Here's how the part is built. I have some questions about the finished solid (model axes, mm). Give positions to 0.01 mm unless a question says otherwise; leave off trailing zeros. Write each loop counter-clockwise with the first axis right and the second up, starting at its lowest first coordinate (ties: lowest second). Pieces come first, ordered by that corner, then holes. Notation, with made-up numbers: (-15, 55) - (33, 55) arc R33 ccw to (33, 85) - close; hole circle Ø7 at (17.5, -35). An arc over 180 degrees is marked (long way). Use a Markdown table: item, result.
```python
from build123d import *

# Parameters (mm, degrees)
EXTRUDE_1_DEPTH     = 5
SKETCH_2_R          = 1.25
CUT_EXTRUDE_1_DEPTH = 5


with BuildPart() as part:
    # 草图1 → 凸台-拉伸1 (new body, symmetric)
    with BuildSketch(Plane(origin=(0, 0, 0), x_dir=(1, 0, 0), z_dir=(0, 1, 0))):
        Polygon((0, -2.598076211), (2.25, -1.299038106), (2.25, 1.299038106), (0, 2.598076211), (-2.25, 1.299038106), (-2.25, -1.299038106), align=None)
    extrude(amount=EXTRUDE_1_DEPTH, both=True)

    # 草图2 → 切除-拉伸1 (cut)
    with BuildSketch(Plane(origin=(0, 5, 0), x_dir=(1, 0, 0), z_dir=(0, 1, 0))):
        Circle(SKETCH_2_R)
    extrude(amount=-CUT_EXTRUDE_1_DEPTH, mode=Mode.SUBTRACT)


solid = part.part
```
Item 1: If we section it at D-D, the plane x = -1.4: Write out the boundary of the cut face in (y, z), plus the area to 3 significant figures.
Values:
| item | result |
|---|---|
| outline | (-5, -1.79) - (5, -1.79) - (5, 1.79) - (-5, 1.79) - close |
| area | 35.8 mm2 |
Item 2: If we section it at B-B, the plane z = -1: Write out the boundary of the cut face in (x, y), plus the area to 3 significant figures.
Values:
| item | result |
|---|---|
| outline | (-2.25, -5) - (2.25, -5) - (2.25, 5) - (0.75, 5) - (0.75, 0) - (-0.75, 0) - (-0.75, 5) - (-2.25, 5) - close |
| area | 37.5 mm2 |
Item 3: I need wall thicknesses on line 1 along X through (y, z) = (2.2, 0); line 2 along X through (y, z) = (3.25, -0.5); line 3 along Y through (x, z) = (-0.45, 0.35). Which ranges of each line are inside material? Lowest first, please. Write a range as [from, to].
Values:
| item | result |
|---|---|
| line 1 | x = [-2.25, -1.25], [1.25, 2.25] |
| line 2 | x = [-2.25, -1.15], [1.15, 2.25] |
| line 3 | y = [-5, 0] |
Item 4: If we section it at C-C, the plane x = 1.15: Write out the boundary of the cut face in (y, z), plus the area to 3 significant figures.
Values:
| item | result |
|---|---|
| outline | (-5, -1.93) - (5, -1.93) - (5, -0.49) - (0, -0.49) - (0, 0.49) - (5, 0.49) - (5, 1.93) - (-5, 1.93) - close |
| area | 33.8 mm2 |
Item 5: Thinking about a two-plate mould opening in Z: for faces 1 (the cylindrical face through (-0.27, 2.54, 1.22)), 2 (the flat face through (0, 0, 0)), 3 (the flat face through (0, -5, 0)), 4 (the flat face through (1.109, 0.07, 1.958)), which applies, +Z half, -Z half, draft (parallel to the pull), parting line (faces both ways), or undercut?
Values:
| item | result |
|---|---|
| face 1 | undercut |
| face 2 | undercut |
| face 3 | draft |
| face 4 | +Z half |
Item 6: If we section it at A-A, the plane y = 3.5: Write out the boundary of the cut face in (x, z).
Values:
| item | result |
|---|---|
| outline | (-2.25, -1.3) - (0, -2.6) - (2.25, -1.3) - (2.25, 1.3) - (0, 2.6) - (-2.25, 1.3) - close; hole circle Ø2.5 at (0, 0) |
